Design review of the part shown in the three views and the two pictorial views. Dimensions are in mm from the part's minimum x, y and z. A direction names the side the tool comes from. Give positions to 0.01 mm unless a question says otherwise; leave off trailing zeros. Loops run counter-clockwise (first coordinate to the right, second up) from the corner with the lowest first, then second, coordinate; pieces in that order, holes last. Notation, with made-up numbers: (57, 62) -> (71, 62) arc R27 ccw to (71, 93) -> close; hole circle Ø11 at (29, 1.5). An arc over 180 degrees is marked (long way). Answer as CSV lines item,"result".
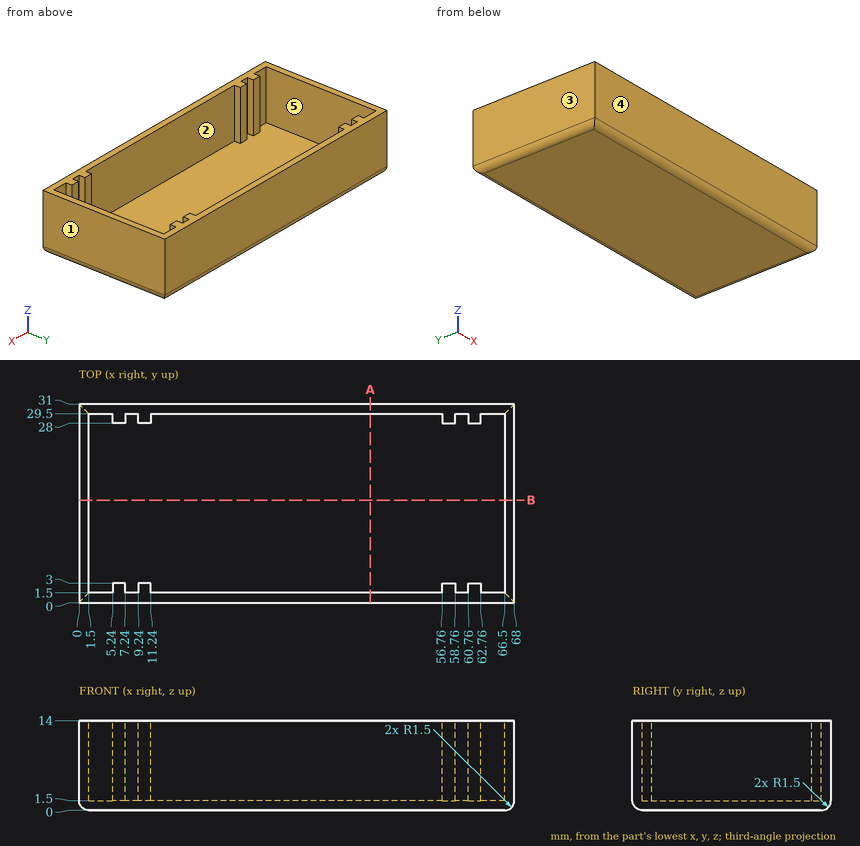
Q1. The part is to be moulded in two halves that separate along X. For the marked faces 1, 2 and 3, say which applies: pulls with the +X half, pulls with the -X half, needs draft (parallel to the pull), parting line crosses it, or undercut.
Filled sheet:
face 1,"pulls with the +X half"
face 2,"undercut"
face 3,"pulls with the -X half"
Q2. For the marked faces 4 and 5, list the 3-axis set-ups (+Z, -Z, +X, -X, +Y, -Y) from which the entire face can be reached by the end or side of a thin tool; tool diameter is ignored.
Filled sheet:
face 4,"+Z, -Z, +X, -X, -Y"
face 5,"+Z"
Q3. Clearance check with a flat-ended pin moving along its axis: pin 1 Ø10 at (x, y) = (7.5, 13) entering from +Z. State where the tip first meets the part, or that it passes through.
Filled sheet:
pin 1,"stops at z = 1.5"
Q4. We need section B-B, the plane y = 16. State the section outline as (x, z) points.
Filled sheet:
outline,"(0, 1.5) arc R1.5 ccw to (1.5, 0) -> (66.5, 0) arc R1.5 ccw to (68, 1.5) -> (68, 14) -> (66.5, 14) -> (66.5, 1.5) -> (1.5, 1.5) -> (1.5, 14) -> (0, 14) -> close"
Q5. To check wall thickness, follow probe 1 along X at (y, z) = (2.5, 6); probe 2 along X at (y, z) = (15.5, 9); probe 3 along Y at (x, z) = (59, 9). State the ranges of each line that lie inside material, in increasing order. Write a range as from..to.
Filled sheet:
probe 1,"x = 0..1.5, 5.24..7.24, 9.24..11.24, 56.76..58.76, 60.76..62.76, 66.5..68"
probe 2,"x = 0..1.5, 66.5..68"
probe 3,"y = 0..1.5, 29.5..31"
Q6. We need section A-A, the plane x = 45.5. State the section outline as (y, z) points.
Filled sheet:
outline,"(0, 1.5) arc R1.5 ccw to (1.5, 0) -> (29.5, 0) arc R1.5 ccw to (31, 1.5) -> (31, 14) -> (29.5, 14) -> (29.5, 1.5) -> (1.5, 1.5) -> (1.5, 14) -> (0, 14) -> close"
